The listing builds one solid part. Answer for the finished solid, in the listing's coordinates (mm). Face numbers are marked on the shaded views. A direction names the side the tool comes from. Coordinates: 2 decimals unless noted, no trailing zeros. Order: outer loops, then holes, each group sorted by start corner. A loop starts at its lowest first (then second) coordinate and runs counter-clockwise, first axis right, second up. Notation, with made-up numbers: (-32.75, 65.25) -> (18.25, 65.25) arc R20 cw to (18.25, 71.25) -> close; hole circle Ø1 at (69, 38.25). An arc over 180 degrees is marked (long way). One line per question, with ' | ' between items.
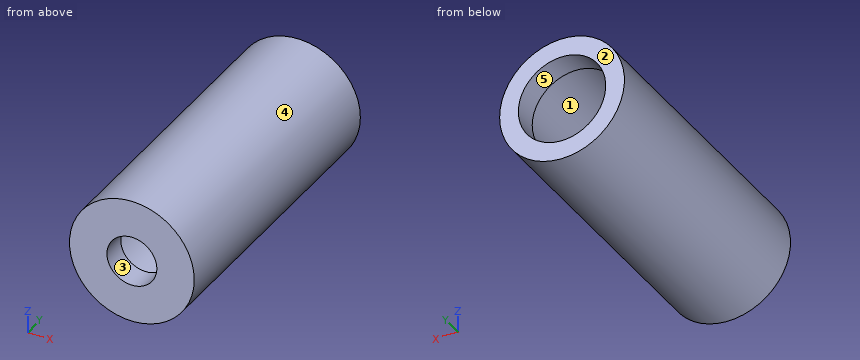
from build123d import *

# Parameters (mm, degrees)
SKETCH1_R           = 25
SKETCH1_R_2         = 20
BOSS_EXTRUDE1_DEPTH = 120
SKETCH2_R           = 20
SKETCH2_R_2         = 17.5
BOSS_EXTRUDE2_DEPTH = 10
SKETCH3_R           = 20
SKETCH3_R_2         = 10
BOSS_EXTRUDE3_DEPTH = 10


with BuildPart() as part:
    # Sketch1 → Boss-Extrude1 (new body)
    with BuildSketch(Plane(origin=(0, 0, 0), x_dir=(1, 0, 0), z_dir=(0, 1, 0))):
        Circle(SKETCH1_R)
        Circle(SKETCH1_R_2, mode=Mode.SUBTRACT)
    extrude(amount=BOSS_EXTRUDE1_DEPTH)

    # Sketch2 → Boss-Extrude2 (add)
    with BuildSketch(Plane(origin=(0, 120, 0), x_dir=(1, 0, 0), z_dir=(0, 1, 0))):
        Circle(SKETCH2_R)
        Circle(SKETCH2_R_2, mode=Mode.SUBTRACT)
    extrude(amount=-BOSS_EXTRUDE2_DEPTH)

    # Sketch3 → Boss-Extrude3 (add)
    with BuildSketch(Plane(origin=(0, 0, 0), x_dir=(-1, 0, 0), z_dir=(0, -1, 0))):
        Circle(SKETCH3_R)
        Circle(SKETCH3_R_2, mode=Mode.SUBTRACT)
    extrude(amount=-BOSS_EXTRUDE3_DEPTH)


solid = part.part
Item 1: Find the intervals of material crossed by L1, parallel to X at y = 112.5, z = 0; L2, parallel to X at y = 6, z = 0, in increasing order.
Computed values:
L1: x = -25 to -17.5, 17.5 to 25 | L2: x = -25 to -10, 10 to 25
Item 2: Section C-C, the plane y = 112.5 is taken. Give the vertices of the cut face in (x, z), plus the area to 3 significant figures.
Computed values:
outline: circle Ø50 at (0, 0); hole circle Ø35 at (0, 0) | area: 1,000 mm^2
Item 3: Each of these flat-tipped pins is pushed along its axis until it touches: pin 1 Ø1 at (y, z) = (25, 9.5) entering from -X; pin 2 Ø12 at (x, y) = (2.5, 46) entering from +Z; pin 3 Ø8 at (x, y) = (2.5, 17.5) entering from -Z; pin 4 Ø21 at (x, z) = (0, 0) entering from -Y. Where does it stop, or does it pass through?
Computed values:
pin 1: stops at x = -23.32 | pin 2: stops at z = 25 | pin 3: stops at z = -25 | pin 4: stops at y = 0
Item 4: Section B-B, the plane x = 0 is taken. Give the vertices of the cut face in (y, z), plus the area to 3 significant figures.
Computed values:
outline: (0, -25) -> (120, -25) -> (120, -17.5) -> (110, -17.5) -> (110, -20) -> (10, -20) -> (10, -10) -> (0, -10) -> close; (0, 10) -> (10, 10) -> (10, 20) -> (110, 20) -> (110, 17.5) -> (120, 17.5) -> (120, 25) -> (0, 25) -> close | area: 1,450 mm^2
Item 5: Determine the mould class of the marked faces 1, 2 and 3 for opening direction Y: pulls with the +Y half, pulls with the -Y half, needs draft (parallel to the pull), parting line crosses it, or undercut.
Computed values:
face 1: undercut | face 2: pulls with the +Y half | face 3: needs draft
Item 6: Section A-A, the plane z = 0 is taken. Give the vertices of the cut face in (x, y).
Computed values:
outline: (-25, 0) -> (-10, 0) -> (-10, 10) -> (-20, 10) -> (-20, 110) -> (-17.5, 110) -> (-17.5, 120) -> (-25, 120) -> close; (10, 0) -> (25, 0) -> (25, 120) -> (17.5, 120) -> (17.5, 110) -> (20, 110) -> (20, 10) -> (10, 10) -> close
Item 7: Section D-D, the plane x = -16 is taken. Give the vertices of the cut face in (y, z), plus the area to 3 significant figures.
Computed values:
outline: (0, -19.21) -> (120, -19.21) -> (120, -7.09) -> (110, -7.09) -> (110, -12) -> (10, -12) -> (10, 12) -> (110, 12) -> (110, 7.09) -> (120, 7.09) -> (120, 19.21) -> (0, 19.21) -> close | area: 2,070 mm^2
Item 8: For the marked faces 4 and 5, determine the directions among +Z, -Z, +X, -X, +Y, -Y from which every point of the face is accessible in a straight line to the end or side of a thin tool.
Computed values:
face 4: +Y, -Y | face 5: +Y
